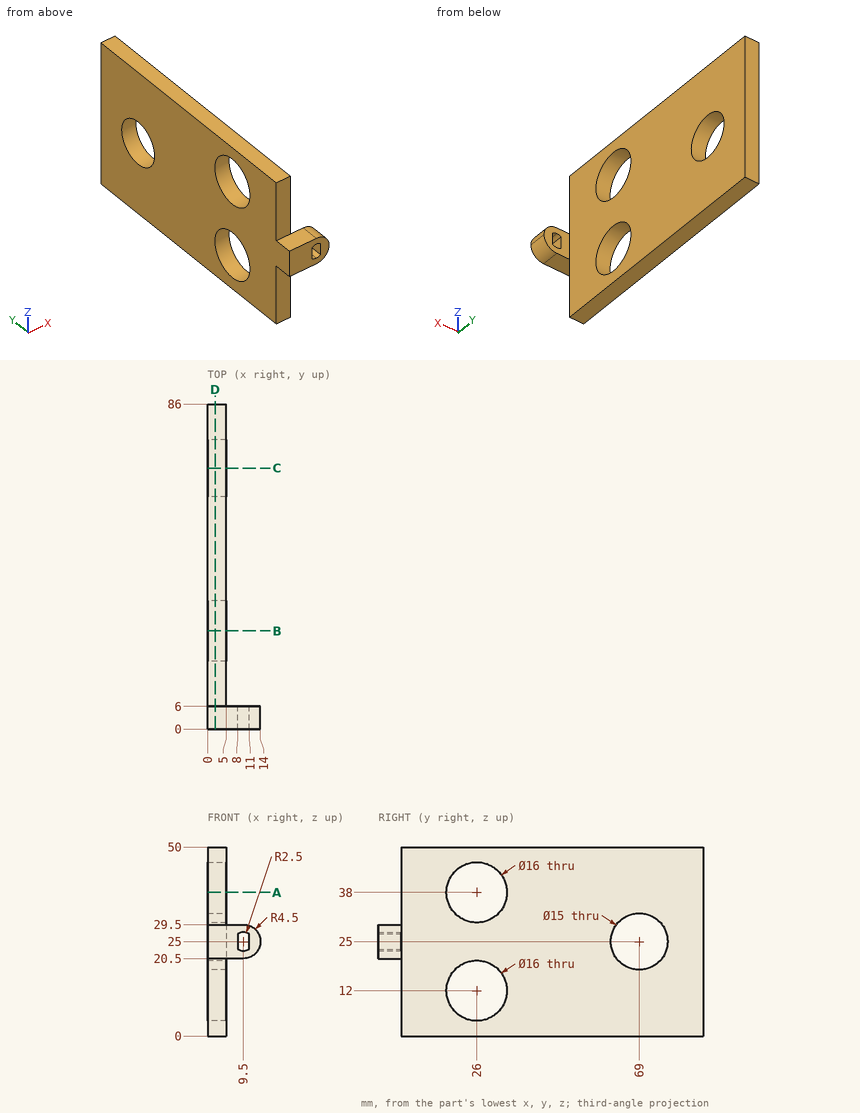
Geometry: see drawing. Coordinates: mm, zero at the bounding-box minimum. Coordinates: 2 decimals unless noted, no trailing zeros. Order: outer loops, then holes, each group sorted by start corner. A loop starts at its lowest first (then second) coordinate and runs counter-clockwise, first axis right, second up. Notation, with made-up numbers: M -36.75,26 L 22.25,26 A15 ccw 22.25,48 Z; hole C 69,87 d10. An arc over 180 degrees is marked long. Write each question's results on one line, items separated by ' | '. Start each with the question number.
1) Section query B-B (y = 26). Return the cut outline in (x, z), plus the area to 3 significant figures.
2) Contact query for flat-ended pins moving along their axis: pin 1 Ø3 at (y, z) = (56, 25.5) entering from +X; pin 2 Ø3 at (x, y) = (3.5, 3) entering from -Z; pin 3 Ø4.5 at (x, z) = (11, 23) entering from +Y. Output: stop coordinate, or through.
3) Section query D-D (x = 2). Return the cut outline in (y, z), plus the area to 3 significant figures.
4) Line query: line 1 (Y direction, x = 2.4, z = 12); line 2 (Y direction, x = 2.8, z = 25); line 3 (X direction, y = 56.5, z = 5). Output: solid intervals per line, ascending. Write a range as from..to.
5) Section query A-A (z = 38). Return the cut outline in (x, y).
6) Section query C-C (y = 69). Return the cut outline in (x, z).
Answers:
1) outline: M 0,0 L 5,0 L 5,4 L 0,4 Z; M 0,20 L 5,20 L 5,30 L 0,30 Z; M 0,46 L 5,46 L 5,50 L 0,50 Z | area: 90.0 mm^2
2) pin 1: stops at x = 5 | pin 2: stops at z = 20.5 | pin 3: stops at y = 6
3) outline: M 0,20.5 L 6,20.5 L 6,0 L 86,0 L 86,50 L 6,50 L 6,29.5 L 0,29.5 Z; hole C 26,12 d16; hole C 26,38 d16; hole C 69,25 d15 | area: 3,480 mm^2
4) line 1: y = 6..18, 34..86 | line 2: y = 0..61.5, 76.5..86 | line 3: x = 0..5
5) outline: M 0,6 L 5,6 L 5,18 L 0,18 Z; M 0,34 L 5,34 L 5,86 L 0,86 Z
6) outline: M 0,0 L 5,0 L 5,17.5 L 0,17.5 Z; M 0,32.5 L 5,32.5 L 5,50 L 0,50 Z
